Could you check a few things on this model? Use its own coordinates, in mm. Face numbers are marked on the shaded views. Round coordinates to 2 decimals unless told otherwise and drop trailing zeros. Write each loop counter-clockwise with the first axis right and the second up, starting at its lowest first coordinate (ties: lowest second). Pieces come first, ordered by that corner, then holes. Notation, with made-up numbers: (84, 44) -> (143, 44) arc R11 cw to (143, 50) -> close; hole circle Ø6 at (24, 19.5). An arc over 180 degrees is marked (long way). Answer in a Markdown table with one row per item.
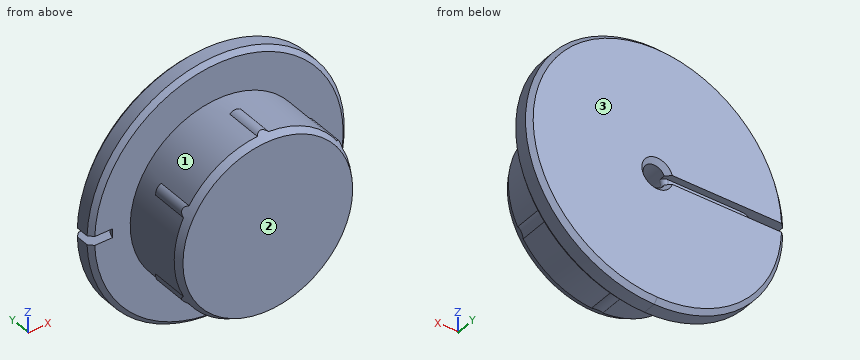
from build123d import *

# Parameters (mm, degrees)
BOSS_EXTRUDE1_START     = -10
BOSS_EXTRUDE1_DEPTH     = 10
CHAMFER1_SIZE           = 1
SKETCH4_W               = 76.07
SKETCH4_H               = 2
CUT_EXTRUDE1_DEPTH      = 46.628938186
CUT_EXTRUDE2_REACH      = 65.581
CUT_EXTRUDE2_END_RADIUS = 2.5
SKETCH5_W               = 2
SKETCH5_H               = 1.5
FILLET1_R               = 4
FILLET2_R               = 1


with BuildPart() as part:
    # Sketch1 → Revolve1 (revolve)
    with BuildSketch(Plane.XY, mode=Mode.PRIVATE) as revolve1_sk:
        Polygon((0, 0), (20, 0), (20, 15), (29, 15), (29, 20), (2.5, 20), (2.5, 10), (0, 10), align=None)
    revolve(revolve1_sk.sketch.rotate(Axis((0, 0, 0), (0, 1, 0)), 90), axis=Axis((0, 0, 0), (0, 1, 0)))

    # Sketch2 → Boss-Extrude1 (add)
    with BuildSketch(Plane.XZ.offset(BOSS_EXTRUDE1_START)):
        with BuildLine():
            ThreePointArc((-1.25, 19.960899278), (0, 20.42), (1.25, 19.960899278))
            ThreePointArc((1.25, 19.960899278), (10, 17.320508076), (16.661645857, 11.062981394))
            ThreePointArc((16.661645857, 11.062981394), (17.684238745, 10.21), (17.911645857, 8.897917884))
            ThreePointArc((17.911645857, 8.897917884), (20, 0), (17.911645857, -8.897917884))
            ThreePointArc((17.911645857, -8.897917884), (17.684238745, -10.21), (16.661645857, -11.062981394))
            ThreePointArc((16.661645857, -11.062981394), (10, -17.320508076), (1.25, -19.960899278))
            ThreePointArc((1.25, -19.960899278), (0, -20.42), (-1.25, -19.960899278))
            ThreePointArc((-1.25, -19.960899278), (-10, -17.320508076), (-16.661645857, -11.062981394))
            ThreePointArc((-16.661645857, -11.062981394), (-17.684238745, -10.21), (-17.911645857, -8.897917884))
            ThreePointArc((-17.911645857, -8.897917884), (-20, 0), (-17.911645857, 8.897917884))
            ThreePointArc((-17.911645857, 8.897917884), (-17.684238745, 10.21), (-16.661645857, 11.062981394))
            ThreePointArc((-16.661645857, 11.062981394), (-10, 17.320508076), (-1.25, 19.960899278))
        make_face()
    extrude(amount=BOSS_EXTRUDE1_DEPTH)

    # Sketch3 → Cut-Revolve1 (revolve, cut)
    with BuildSketch(Plane.XY, mode=Mode.PRIVATE) as cut_revolve1_sk:
        Polygon((-21, 3.232050808), (-18.556624327, -1), (-21, -1), align=None)
    revolve(cut_revolve1_sk.sketch.rotate(Axis((0, 29.336873575, 0), (0, -1, 0)), 273.58332148), axis=Axis((0, 29.336873575, 0), (0, -1, 0)), mode=Mode.SUBTRACT)

    # Chamfer1
    chamfer1_edges = [part.edges().sort_by_distance(p)[0] for p in [
        (0, 20, 2.5),
        (0, 20, 29),
        (0, 15, 29),
    ]]
    chamfer(chamfer1_edges, length=CHAMFER1_SIZE)

    # Sketch4 → Cut-Extrude1 (cut, through all)
    with BuildSketch(Plane.XZ):
        with Locations((-61.965, 0)):
            Rectangle(SKETCH4_W, SKETCH4_H)
    extrude(amount=-CUT_EXTRUDE1_DEPTH, mode=Mode.SUBTRACT)

    # Cut-Extrude2: up to this cylinder (the profile starts outside it)
    cut_extrude2_end = Plane(origin=(0, 19.25, 0), z_dir=(0, -1, 0)) * Cylinder(CUT_EXTRUDE2_END_RADIUS, 137.162, mode=Mode.PRIVATE)
    # Sketch5 → Cut-Extrude2 (cut, up to the surface)
    with BuildSketch(Plane.ZY.offset(23.93), mode=Mode.PRIVATE) as cut_extrude2_sk1:
        with Locations((0, 19.25)):
            Rectangle(SKETCH5_W, SKETCH5_H)
    cut_extrude2_tool1 = extrude(cut_extrude2_sk1.sketch, amount=-CUT_EXTRUDE2_REACH, mode=Mode.PRIVATE) - cut_extrude2_end
    add(cut_extrude2_tool1.solids().sort_by_distance((-23.93, 19.25, 0))[0], mode=Mode.SUBTRACT)

    # Fillet1
    # the kernel refuses this fillet: 4 mm, written as the material it takes off along each edge
    with BuildSketch(Plane(origin=(-23.93, 18.5, 1), x_dir=(1, 0, 0), z_dir=(0, 0, -1))) as fillet1_piece_1:
        with BuildLine():
            CenterArc((3.968626967, 4), FILLET1_R, 187.180755781, 82.819244219)
            Line((0, 3.5), (-0.079372539, 3.49))
            ThreePointArc((-0.079372539, 3.49), (-0.08, 1.75), (-0.08, 0))
            Line((-0.08, 0), (0, -0.08))
            Line((0, -0.08), (3.968626967, -0.08))
            Line((3.968626967, -0.08), (3.968626967, 0))
        make_face()
    extrude(amount=2, mode=Mode.SUBTRACT)

    # Fillet2
    fillet2_edges = [part.edges().sort_by_distance(p)[0] for p in [
        (-2.5, 18.5, 0),
    ]]
    fillet(fillet2_edges, radius=FILLET2_R)


solid = part.part
1) For pin 1 (4 mm diameter, centred on x = 10, z = -20, fed in from -Y); pin 2 (3 mm diameter, centred on y = 16, z = 11, fed in from -X); pin 3 (1 mm diameter, centred on y = 6, z = -11, fed in from -X), each with a flat end and sliding along its axis, tell me the tip position at first contact or that it passes through.
Findings:
| item | result |
|---|---|
| pin 1 | stops at y = 15 |
| pin 2 | stops at x = -27.4 |
| pin 3 | stops at x = -17.48 |
2) Imagine slicing it at A-A, the plane z = 0. Please give me the cut outline in (x, y).
Findings:
| item | result |
|---|---|
| outline | (-23.93, 15) -> (-20, 15) -> (-20, 1.5) -> (-19.13, 0) -> (19.13, 0) -> (20, 1.5) -> (20, 15) -> (28, 15) -> (29, 16) -> (29, 19) -> (28, 20) -> (3.5, 20) -> (2.5, 19) -> (2.5, 10) -> (-2.5, 10) -> (-2.5, 17.5) arc R1 ccw to (-3.5, 18.5) -> (-19.96, 18.5) arc R4 ccw to start |
3) Imagine slicing it at C-C, the plane y = 8.5. Please give me the cut outline in (x, z).
Findings:
| item | result |
|---|---|
| outline | (-17.91, -8.9) arc R1.93 ccw to (-16.66, -11.06) arc R20 ccw to (-1.25, -19.96) arc R1.93 ccw to (1.25, -19.96) arc R20 ccw to (16.66, -11.06) arc R1.93 ccw to (17.91, -8.9) arc R20 ccw to (17.91, 8.9) arc R1.93 ccw to (16.66, 11.06) arc R20 ccw to (1.25, 19.96) arc R1.93 ccw to (-1.25, 19.96) arc R20 ccw to (-16.66, 11.06) arc R1.93 ccw to (-17.91, 8.9) arc R20 ccw to start |
4) Thinking about a two-plate mould opening in Y: for the marked faces 1, 2 and 3, which applies, +Y half, -Y half, draft (parallel to the pull), parting line (faces both ways), or undercut?
Findings:
| item | result |
|---|---|
| face 1 | undercut |
| face 2 | -Y half |
| face 3 | +Y half |
5) Imagine slicing it at B-B, the plane y = 11.75. Please give me the cut outline in (x, z), plus the area to 3 significant figures.
Findings:
| item | result |
|---|---|
| outline | circle Ø40 at (0, 0); hole circle Ø5 at (0, 0) |
| area | 1,240 mm^2 |
6) Please list where these lines run through material, in increasing order: line 1 (X direction, y = 13.5, z = 0); line 2 (Y direction, x = -3.5, z = 23); line 3 (X direction, y = 15.25, z = 0).
Findings:
| item | result |
|---|---|
| line 1 | x = -20 to -2.5, 2.5 to 20 |
| line 2 | y = 15 to 20 |
| line 3 | x = -23.89 to -2.5, 2.5 to 28.25 |
